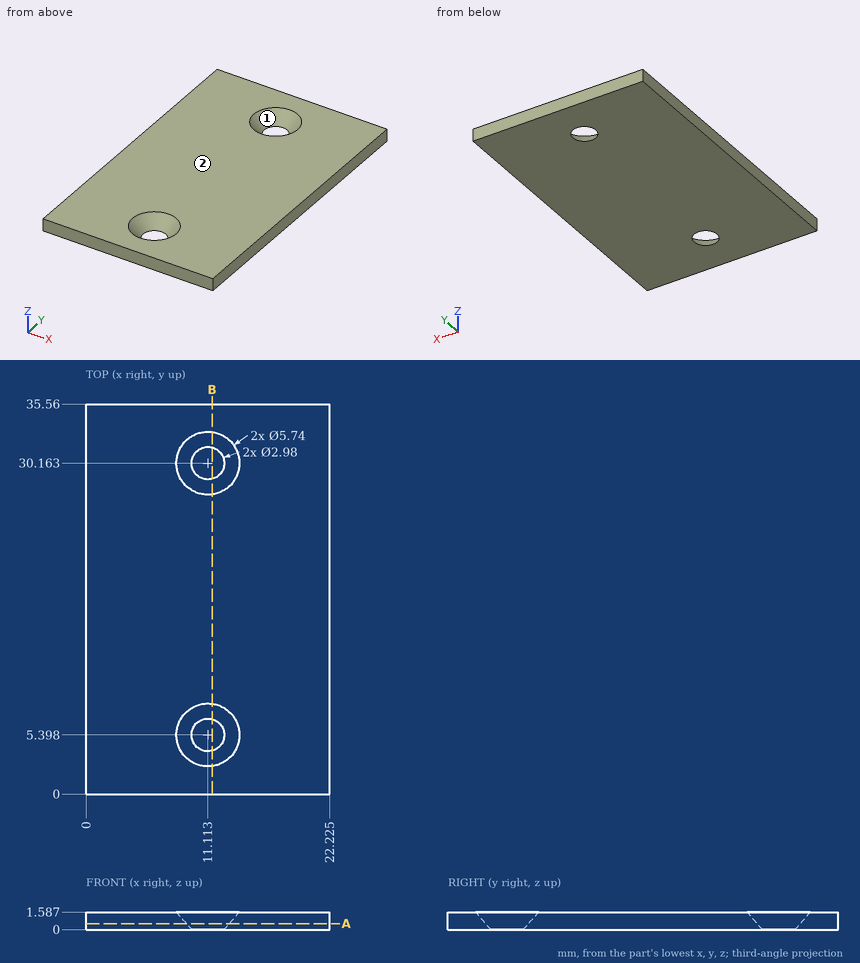
The figure shows three views and two pictorial views of one solid part (mm, origin at its lowest corner). Answer the questions. Give positions to 0.01 mm unless a question says otherwise; leave off trailing zeros. Write each loop counter-clockwise with the first axis right and the second up, starting at its lowest first coordinate (ties: lowest second). Pieces come first, ordered by that corner, then holes. Notation, with made-up numbers: (51, 81.5) - (96, 81.5) arc R32 cw to (96, 110.5) - close; hole circle Ø6 at (-5, 83.5). An arc over 180 degrees is marked (long way). Use one line per item in the form item = value.
1. A cutting plane is placed at A-A (z = 0.55). Write down the section's boundary in (x, y) (1 decimal).
Filled in:
outline = (0, 0) - (22.2, 0) - (22.2, 35.6) - (0, 35.6) - close; hole circle Ø3.9 at (11.1, 5.4); hole circle Ø3.9 at (11.1, 30.2)
2. A cutting plane is placed at B-B (x = 11.5). State how many separate pieces and enclosed holes the cut face has.
Filled in:
separate_pieces = 3
enclosed_holes = 0
3. Consider L1, parallel to X at y = 30, z = 1.15 (1 decimal); L2, parallel to X at y = 30, z = 1.45 (1 decimal); L3, parallel to Z at x = 9, y = 29. Determine where each line is inside the solid, lowest interval first.
Filled in:
L1 = 0 to 8.6, 13.6 to 22.2
L2 = 0 to 8.4, 13.9 to 22.2
L3 = 0 to 1.06
4. Determine the mould class of the marked faces 1 and 2 for opening direction Y: released by +Y, released by -Y, zero draft, split by the parting line, or undercut.
Filled in:
face_1 = undercut
face_2 = zero draft
